Can you work these out from the model? Positions are in its coordinate system, mm. Face numbers are marked on the shaded views. A direction names the side the tool comes from. Round coordinates to 2 decimals unless told otherwise and drop trailing zeros. Loops run counter-clockwise (first coordinate to the right, second up) from the corner with the lowest first, then second, coordinate; pieces in that order, holes last. Notation, with made-up numbers: M 66,19.25 L 118,19.25 A19 cw 118,32.25 Z; hole C -19,62 d9. An arc over 180 degrees is marked long. Return JSON: item names as keys, results as strings.
```python
from build123d import *

# Parameters (mm, degrees)
SKETCH1_R           = 14.224
BOSS_EXTRUDE1_DEPTH = 6.35
ONEHOLE_START       = -0.1524
SKETCH2_R           = 2.4892
ONEHOLE_DEPTH       = 0.1524


with BuildPart() as part:
    # Sketch1 → Boss-Extrude1 (new body, symmetric)
    with BuildSketch(Plane(origin=(0, 0, 0), x_dir=(0, 0, -1), z_dir=(1, 0, 0))):
        with BuildLine():
            Line((0, 15.494), (50.8, 15.494))
            Line((50.8, 15.494), (50.8, 15.3416))
            Line((50.8, 15.3416), (2.167797371, 15.3416))
            ThreePointArc((2.167797371, 15.3416), (-1.086573882, -15.45585304), (0, 15.494))
        make_face()
        Circle(SKETCH1_R, mode=Mode.SUBTRACT)
    extrude(amount=BOSS_EXTRUDE1_DEPTH, both=True)

    # Sketch2 → OneHole (cut)
    with BuildSketch(Plane(origin=(0, 15.494, 0), x_dir=(1, 0, 0), z_dir=(0, 1, 0)).offset(ONEHOLE_START)):
        with Locations((0, 42.0878)):
            Circle(SKETCH2_R)
        with BuildLine():
            Line((-6.35, 49.710512242), (-6.35, 51.435))
            Line((-6.35, 51.435), (6.35, 51.435))
            Line((6.35, 51.435), (6.35, 49.710512242))
            ThreePointArc((6.35, 49.710512242), (0, 50.8), (-6.35, 49.710512242))
        make_face()
    extrude(amount=ONEHOLE_DEPTH, mode=Mode.SUBTRACT)


solid = part.part
```
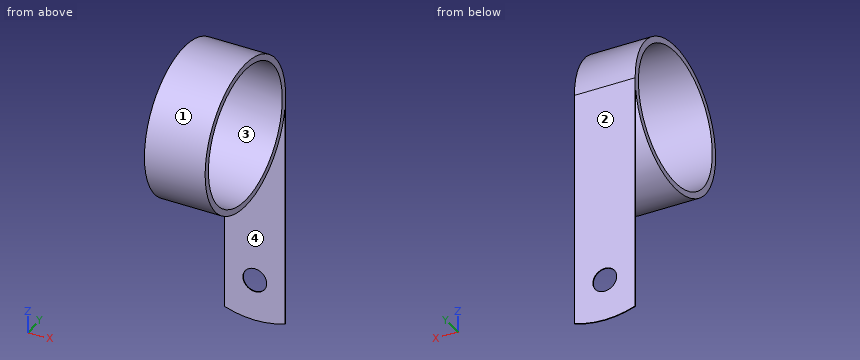
Q1. Suppose I cut it at B-B, the plane x = 0. Please give me the cut outline in (y, z).
Results:
{"outline": "M 15.34,-50.8 L 15.49,-50.8 L 15.49,-44.58 L 15.34,-44.58 Z; M 15.34,-39.6 L 15.49,-39.6 L 15.49,0 A15.49 ccw long 15.34,-2.17 Z; hole C 0,0 d28.45"}
Q2. Suppose I cut it at D-D, the plane x = 5. Please give me the cut outline in (y, z).
Results:
{"outline": "M 15.34,-50.13 L 15.49,-50.13 L 15.49,0 A15.49 ccw long 15.34,-2.17 Z; hole C 0,0 d28.45"}
Q3. I'm going to push flat-ended pins straight in: pin 1 Ø3 at (x, y) = (1.5, 4) entering from +Z; pin 2 Ø5.5 at (x, z) = (0, -42.09) entering from -Y. Where does each tip first touch, or does it pass through?
Results:
{"pin 1": "stops at z = 15.29", "pin 2": "stops at y = 15.34"}
Q4. Suppose I cut it at A-A, the plane y = 0. Please give me the cut outline in (x, z), plus the area to 3 significant figures.
Results:
{"outline": "M -6.35,-15.49 L 6.35,-15.49 L 6.35,-14.22 L -6.35,-14.22 Z; M -6.35,14.22 L 6.35,14.22 L 6.35,15.49 L -6.35,15.49 Z", "area": "32.3 mm2"}
Q5. Suppose I cut it at C-C, the plane z = -13. Please give me the cut outline in (x, y), plus the area to 3 significant figures.
Results:
{"outline": "M -6.35,-8.43 L 6.35,-8.43 L 6.35,-5.77 L -6.35,-5.77 Z; M -6.35,5.77 L 6.35,5.77 L 6.35,8.43 L -6.35,8.43 Z; M -6.35,15.34 L 6.35,15.34 L 6.35,15.49 L -6.35,15.49 Z", "area": "69.4 mm2"}
Q6. Thinking about a two-plate mould opening in Y: for the marked faces 1 and 2, which applies, pulls with the +Y half, pulls with the -Y half, needs draft (parallel to the pull), parting line crosses it, or undercut?
Results:
{"face 1": "undercut", "face 2": "pulls with the +Y half"}
Q7. If I drill on line 1 along Z through (x, y) = (3.5, -0.5); line 2 along Y through (x, z) = (0.5, -16); line 3 along Z through (x, y) = (3.25, -6.5), over which ranges is the centre line in solid material (lowest first)?
Results:
{"line 1": "z = -15.49 to -14.22, 14.22 to 15.49", "line 2": "y = 15.34 to 15.49", "line 3": "z = -14.06 to -12.65, 12.65 to 14.06"}
Q8. On a 3-axis mill with a long thin cutter (end or side, diameter ignored), from which of +Z, -Z, +X, -X, +Y, -Y can I reach the whole of each face in a straight line? I mean the marked faces 3 and 4. Say none if no direction works.
Results:
{"face 3": "+X, -X", "face 4": "-Z, +X, -X"}
